Verification items for the finished model (mm, model axes). Face numbers are marked on the shaded views. A direction names the side the tool comes from. Round coordinates to 2 decimals unless told otherwise and drop trailing zeros. Order: outer loops, then holes, each group sorted by start corner. A loop starts at its lowest first (then second) coordinate and runs counter-clockwise, first axis right, second up. Notation, with made-up numbers: (-9, 15.25) -> (34, 15.25) arc R17 cw to (34, 22.25) -> close; hole circle Ø4 at (42, -4). An arc over 180 degrees is marked (long way). Put each result on its own line as item: value.
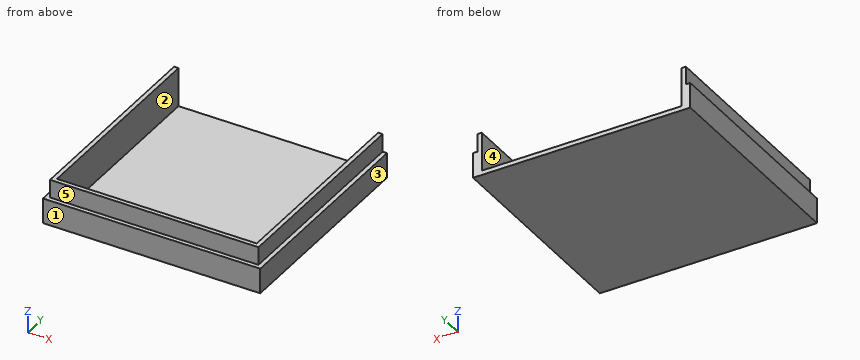
Autodesk Inventor part; units mm, degrees
ref_plane "YZ Plane" through (0, 0, 0) normal (1, 0, 0) x (0, 1, 0)
ref_plane "XZ Plane" through (0, 0, 0) normal (0, 1, 0) x (-1, 0, 0)
ref_plane "XY Plane" through (0, 0, 0) normal (0, 0, 1) x (1, 0, 0)
sketch "Sketch1" plane through (0, 0, 0) normal (0, 1, 0) x (-1, 0, 0)
  line L0 (0, 0) -> (95.25, 0)
  line L1 (95.25, 0) -> (95.25, -9.525)
  line L2 (95.25, -9.525) -> (0, -9.525)
  line L3 (0, -9.525) -> (0, 0)
  line L4 (-2, -11.525) -> (97.25, -11.525)
  line L5 (97.25, -11.525) -> (97.25, 2)
  line L6 (97.25, 2) -> (-2, 2)
  line L7 (-2, 2) -> (-2, -11.525)
  line L8 (95.25, 0) -> (97.25, 0)
  line L9 (0, 0) -> (-2, 0)
  dimension "d0" = 95.25
  dimension "d1" = 9.525
  dimension "d4" = 2
extrude "Extrusion1" add sketch "Sketch1" along normal blind 2 contours L0 L1 L2 L3 | L3 L2 L1 L8 L5 L4 L7 L9
sketch "Sketch2" plane through (0, 2, 0) normal (0, 1, 0) x (1, 0, 0)
  line L0 (-97.25, 0) -> (2, 0)
  line L1 (2, 0) -> (2, 11.525)
  line L2 (2, 11.525) -> (-97.25, 11.525)
  line L3 (-97.25, 11.525) -> (-97.25, 0)
  line L4 (0, 9.525) -> (0, 2)
  line L5 (0, 2) -> (-95.25, 2)
  line L6 (-95.25, 2) -> (-95.25, 9.525)
  line L7 (-95.25, 9.525) -> (0, 9.525)
  line L8 (0, 2) -> (0, 0)
  line L9 (-95.25, 2) -> (-95.25, 0)
  dimension "d5" = 2
extrude "Extrusion2" add sketch "Sketch2" along normal blind 95.25 contours L3 L2 L1 L0 L8 L4 L7 L6 L9
sketch "Sketch4" plane through (-95.25, 2, -9.525) normal (0, 0, 1) x (1, 0, 0)
  line L0 (95.25, 0) -> (0, 0)
  line L1 (95.25, 0) -> (95.25, 95.25)
  line L2 (0, 95.25) -> (95.25, 95.25)
  line L3 (0, 0) -> (0, 95.25)
  line L4 (2, 93.25) -> (93.25, 93.25)
  line L5 (93.25, 93.25) -> (93.25, 2)
  line L6 (93.25, 2) -> (2, 2)
  line L7 (2, 2) -> (2, 93.25)
  line L8 (2, 93.25) -> (93.25, 93.25)
  line L9 (93.25, 93.25) -> (93.25, 95.25)
  line L10 (93.25, 95.25) -> (2, 95.25)
  line L11 (2, 95.25) -> (2, 93.25)
  point P0 (95.25, -2)
  point P1 (2, 95.25)
  dimension "d11" = 2
extrude "Extrusion4" add sketch "Sketch4" along normal blind 17.78 contours L0 L3 L2 L11 L7 L6 L5 L9 L1
properties part number "front"
Item 1: Sectioned sample at B-B, the plane z = 3. Record the boundary of the cut face in (x, y).
Geometry check:
outline: (-95.25, 2) -> (0, 2) -> (0, 97.25) -> (-2, 97.25) -> (-2, 4) -> (-93.25, 4) -> (-93.25, 97.25) -> (-95.25, 97.25) -> close
Item 2: Sectioned sample at A-A, the plane y = 43. Record the boundary of the cut face in (x, z) (3 decimals), then the cut area to 3 significant figures.
Geometry check:
outline: (-97.25, -11.525) -> (2, -11.525) -> (2, 0) -> (0, 0) -> (0, 8.255) -> (-2, 8.255) -> (-2, -9.525) -> (-93.25, -9.525) -> (-93.25, 8.255) -> (-95.25, 8.255) -> (-95.25, 0) -> (-97.25, 0) -> close
area: 308 mm2
Item 3: Sectioned sample at C-C, the plane x = -57.5. Record the boundary of the cut face in (y, z) (3 decimals), then the cut area to 3 significant figures.
Geometry check:
outline: (0, -11.525) -> (97.25, -11.525) -> (97.25, -9.525) -> (4, -9.525) -> (4, 8.255) -> (2, 8.255) -> (2, 0) -> (0, 0) -> close
area: 249 mm2
Item 4: Depth check by flat-ended pin: pin 1 Ø3 at (y, z) = (39.5, 2) entering from +X; pin 2 Ø2 at (y, z) = (84, 0.5) entering from +X; pin 3 Ø10 at (x, z) = (-11, 3) entering from +Y; pin 4 Ø6.5 at (x, z) = (-31.5, 6) entering from -Y. Enter the tip coordinate at first touch or a pass-through.
Geometry check:
pin 1: x = 0
pin 2: x = 2
pin 3: y = 4
pin 4: y = 2
Item 5: Tool access check on the marked faces 1 and 2. Record the directions out of +Z, -Z, +X, -X, +Y, -Y that give a thin tool (end or side, any length) a straight path to the whole face; none if there is none.
Geometry check:
face 1: +Z, -Z, +X, -X, -Y
face 2: +Z, +Y
Item 6: Material ranges on line 1 along X through (y, z) = (79.5, -2.5); line 2 along X through (y, z) = (10, 1.75); line 3 along Z through (x, y) = (-14, 49) (3 decimals), recorded low to high.
Geometry check:
line 1: -97.25 to -93.25, -2 to 2
line 2: -95.25 to -93.25, -2 to 0
line 3: -11.525 to -9.525
Item 7: Release check for a two-part mould opening along X. For the marked faces 3, 4 and 5 record: pulls with the +X half, pulls with the -X half, needs draft (parallel to the pull), parting line crosses it, or undercut.
Geometry check:
face 3: pulls with the +X half
face 4: undercut
face 5: needs draft
